```python
from build123d import *

# Parameters (mm, degrees)
F0_W     = 169
F0_H     = 104
F1_DEPTH = 5.6
F2_W     = 158.5
F2_H     = 90.5
F3_DEPTH = 0.1
F4_R     = 2
F4_R_2   = 1.5
F5_DEPTH = 4.4


with BuildPart() as f1:
    # F0 (on Top) → F1 (new body)
    with BuildSketch(Plane.XY):
        with Locations((84.5, 52)):
            Rectangle(F0_W, F0_H)
    extrude(amount=F1_DEPTH)

    # F2 (on face) → F3 (cut)
    with BuildSketch(Plane.XY.offset(5.6)):
        with Locations((82.35, 55.65)):
            Rectangle(F2_W, F2_H)
    extrude(amount=-F3_DEPTH, mode=Mode.SUBTRACT)

    # F4 (on face) → F5 (join)
    with BuildSketch(Plane(origin=(0, 0, 0), x_dir=(1, 0, 0), z_dir=(0, 0, -1))):
        with Locations((163.1, -97.1)):
            Circle(F4_R)
        with Locations((163.1, -97.1)):
            Circle(F4_R_2, mode=Mode.SUBTRACT)
        with Locations((5.9, -97.1)):
            Circle(F4_R)
        with Locations((5.9, -97.1)):
            Circle(F4_R_2, mode=Mode.SUBTRACT)
        with Locations((5.9, -6.9)):
            Circle(F4_R)
        with Locations((5.9, -6.9)):
            Circle(F4_R_2, mode=Mode.SUBTRACT)
        with Locations((163.1, -6.9)):
            Circle(F4_R)
        with Locations((163.1, -6.9)):
            Circle(F4_R_2, mode=Mode.SUBTRACT)
    extrude(amount=F5_DEPTH)


solid = f1.part
```
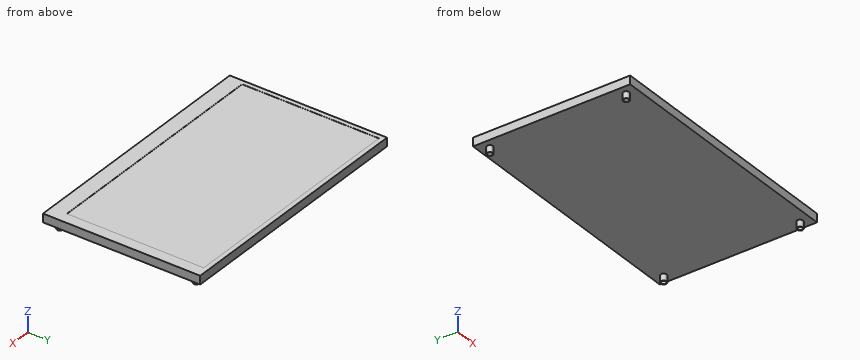
Model file for the job. Use its own axes, mm. Give positions to 0.01 mm unless a question says otherwise; leave off trailing zeros. Loops run counter-clockwise (first coordinate to the right, second up) from the corner with the lowest first, then second, coordinate; pieces in that order, holes last. Notation, with made-up numbers: (2.25, -13.5) - (46.25, -13.5) arc R17 cw to (46.25, 7.5) - close; hole circle Ø7 at (-12, 44.25). An arc over 180 degrees is marked (long way). One line per item, written item: value. Start each with the question number.
1. Slice it at B-B (y = 29). List the corners of the cut face in (x, z).
2. Probe L1, parallel to Y at x = 163.1, z = -3.15; L2, parallel to X at y = 6.9, z = -1.45; L3, parallel to Z at x = 87, y = 46.5. List the from-to ranges inside material, lowest first. Write a range as from..to.
3. Pin check, flat tips, straight feed: pin 1 (1.8 mm diameter, centred on x = 163.1, y = 6.9, fed in from -Z); pin 2 (2.5 mm diameter, centred on x = 5.9, y = 97.1, fed in from +Z); pin 3 (1.5 mm diameter, centred on y = 57, z = -1.5, fed in from -X). Stop position of each tip, or through.
4. Slice it at A-A (z = -1.75). List the corners of the cut face in (x, y), plus the area to 3 significant figures.
5. Slice it at C-C (x = 21). List the corners of the cut face in (y, z).
Solution:
1. outline: (0, 0) - (169, 0) - (169, 5.6) - (161.6, 5.6) - (161.6, 5.5) - (3.1, 5.5) - (3.1, 5.6) - (0, 5.6) - close
2. L1: y = 4.9..5.4, 8.4..8.9, 95.1..95.6, 98.6..99.1
2. L2: x = 3.9..4.4, 7.4..7.9, 161.1..161.6, 164.6..165.1
2. L3: z = 0..5.5
3. pin 1: stops at z = 0
3. pin 2: stops at z = 5.5
3. pin 3: passes through
4. outline: circle Ø4 at (5.9, 6.9); circle Ø4 at (5.9, 97.1); circle Ø4 at (163.1, 6.9); circle Ø4 at (163.1, 97.1); hole circle Ø3 at (5.9, 6.9); hole circle Ø3 at (5.9, 97.1); hole circle Ø3 at (163.1, 6.9); hole circle Ø3 at (163.1, 97.1)
4. area: 22.0 mm^2
5. outline: (0, 0) - (104, 0) - (104, 5.6) - (100.9, 5.6) - (100.9, 5.5) - (10.4, 5.5) - (10.4, 5.6) - (0, 5.6) - close
